Autodesk Inventor part; units mm, degrees
ref_plane "YZ Plane" through (0, 0, 0) normal (1, 0, 0) x (0, 1, 0)
ref_plane "XZ Plane" through (0, 0, 0) normal (0, 1, 0) x (-1, 0, 0)
ref_plane "XY Plane" through (0, 0, 0) normal (0, 0, 1) x (1, 0, 0)
sketch "スケッチ1" plane through (0, 0, 0) normal (0, 1, 0) x (-1, 0, 0)
  line L0 (0, 0) -> (-5, 0)
  line L1 (-5, 0) -> (-5, 2.8)
  line L2 (-5, 2.8) -> (-3, 2.8)
  line L3 (-3, 2.8) -> (-3, 7.3)
  line L4 (-3, 7.3) -> (-2, 7.3)
  line L5 (-2, 7.3) -> (-2, 11.87)
  line L6 (-1.57, 12.3) -> (0, 12.3)
  line L7 (0, 12.3) -> (0, 0)
  line L8 (-1.57, 12.3) -> (-2, 11.87)
  point P0 (-2, 12.3)
  dimension "d0" = 5
  dimension "d1" = 4.5
  dimension "d2" = 2.8
  dimension "d3" = 0.43
  dimension "d4" = 0.43
  dimension "d5" = 4
  dimension "d6" = 10
  dimension "d7" = 6
revolve "回転1" add sketch "スケッチ1" angle 360 about axis through (0, 0, 12.3) along (0, 0, -1)
thread "ねじ1"
sketch "スケッチ2" plane through (0, 0, 0) normal (0, 0, -1) x (-1, 0, 0)
  line L0 (0, -1.4434) -> (-1.25, -0.7217)
  line L1 (-1.25, -0.7217) -> (-1.25, 0.7217)
  line L2 (-1.25, 0.7217) -> (0, 1.4434)
  line L3 (0, 1.4434) -> (1.25, 0.7217)
  line L4 (1.25, 0.7217) -> (1.25, -0.7217)
  line L5 (1.25, -0.7217) -> (0, -1.4434)
  point P0 (0, 0)
  point P1 (0, 0)
  dimension "d11" = 2.5
extrude "押し出し1" cut sketch "スケッチ2" against normal blind 1.5
sketch "スケッチ3" plane through (0, 0, 12.3) normal (0, 0, 1) x (1, 0, 0)
  circle A0 centre (0, 0) radius 2
extrude "押し出し2" cut sketch "スケッチ3" against normal blind 2
properties part number "DBTS4-4.5-5-DHC-LTC_mod" material "ステンレス鋼 AISI 304"
Could you check a few things on this model? Use its own coordinates, in mm. A direction names the side the tool comes from. Round coordinates to 2 decimals unless told otherwise and drop trailing zeros. Loops run counter-clockwise (first coordinate to the right, second up) from the corner with the lowest first, then second, coordinate; pieces in that order, holes last. Notation, with made-up numbers: M 16,76.25 L 71,76.25 A25 cw 71,93.25 Z; hole C 40.5,-31 d1. An arc over 180 degrees is marked long. Answer as CSV lines item,"result".
1) For pin 1 Ø6 at (x, z) = (-3.5, 7.5) entering from -Y; pin 2 Ø1.5 at (y, z) = (0.5, 2.5) entering from +X; pin 3 Ø1 at (y, z) = (-2.5, 1.5) entering from -X; pin 4 Ø1 at (x, z) = (-3, 7) entering from +Y, each with a flat end and sliding along its axis, tell me the tip position at first contact or that it passes through.
From the geometry:
pin 1,"y = -2.96"
pin 2,"x = 5"
pin 3,"x = -4.58"
pin 4,"y = 1.66"
2) If I drill on probe 1 along Z at (x, y) = (3.75, -3); probe 2 along Z at (x, y) = (1.5, 2.25); probe 3 along X at (y, z) = (-2.5, 4), over which ranges is the centre line in solid material (lowest first)?
From the geometry:
probe 1,"0 to 2.8"
probe 2,"0 to 7.3"
probe 3,"-1.66 to 1.66"
3) Imagine slicing it at A-A on y = 0. List the corners of the cut face in (x, z) for me.
From the geometry:
outline,"M -5,0 L -1.25,0 L -1.25,1.5 L 1.25,1.5 L 1.25,0 L 5,0 L 5,2.8 L 3,2.8 L 3,7.3 L 2,7.3 L 2,10.3 L -2,10.3 L -2,7.3 L -3,7.3 L -3,2.8 L -5,2.8 Z"
4) We'd pull the mould along Y, two halves only. Please class faces 1 (the cylindrical face through (0, -2, 9)), 2 (the flat face through (3.3, -0.1, 2.8)), 3 (the flat face through (0.63, 1.08, 0.74)): released by +Y, released by -Y, zero draft, split by the parting line, or undercut.
From the geometry:
face 1,"split by the parting line"
face 2,"zero draft"
face 3,"undercut"
5) Which directions (+Z, -Z, +X, -X, +Y, -Y) give clear straight access to the entire face, cutting with the end or side of a thin tool? Please do faces 4 (the flat face through (0, 0, 10.3)), 5 (the flat face through (1, 2, 7.3)), 6 (the flat face through (-1.25, 0, 1)).
From the geometry:
face 4,"+Z, +X, -X, +Y, -Y"
face 5,"+Z"
face 6,"-Z"
6) Imagine slicing it at C-C on z = 9. List the corners of the cut face in (x, y) for me, and give its area (3 significant figures).
From the geometry:
outline,"C 0,0 d4"
area,"12.6 mm^2"
7) Imagine slicing it at B-B on x = -0.25. List the corners of the cut face in (y, z) for me, and give its area (3 significant figures).
From the geometry:
outline,"M -4.99,0 L -1.3,0 L -1.3,1.5 L 1.3,1.5 L 1.3,0 L 4.99,0 L 4.99,2.8 L 2.99,2.8 L 2.99,7.3 L 1.98,7.3 L 1.98,10.3 L -1.98,10.3 L -1.98,7.3 L -2.99,7.3 L -2.99,2.8 L -4.99,2.8 Z"
area,"62.9 mm^2"
8) Imagine slicing it at D-D on y = -2.75. List the corners of the cut face in (x, z) for me, and give its area (3 significant figures).
From the geometry:
outline,"M -4.18,0 L 4.18,0 L 4.18,2.8 L 1.2,2.8 L 1.2,7.3 L -1.2,7.3 L -1.2,2.8 L -4.18,2.8 Z"
area,"34.2 mm^2"
